```python
from build123d import *

# Parameters (mm, degrees)
SKETCH_1_W                       = 52
SKETCH_1_H                       = 25
SM_BASE_FLANGE_1_DEPTH           = 2
SM_EDGE_FLANGE_1_STRIP_W         = 9.4732
SM_EDGE_FLANGE_1_STRIP_H         = 2
SM_EDGE_FLANGE_1_STRIP_CUT_DEPTH = 25
SM_EDGE_FLANGE_1_DEPTH           = 25
SM_START                         = 2
SM_EDGE_FLANGE_1_FLAT_DEPTH      = 2
HOLE_WIZARD_3_0_3_1_D            = 3
HOLE_WIZARD_8_0_8_2_D            = 8
HOLE_WIZARD_8_0_8_3_D            = 8
HOLE_WIZARD_3_0_3_2_D            = 3


# Sheet-metal steps are written as plain solids
with BuildPart() as part:
    # Sketch 1 → 基体-法兰1 (new body)
    with BuildSketch(Plane(origin=(0, 0, 0), x_dir=(1, 0, 0), z_dir=(0, 1, 0))):
        Rectangle(SKETCH_1_W, SKETCH_1_H)
    extrude(amount=-SM_BASE_FLANGE_1_DEPTH)

    # 边线-法兰1 strip (across the edge) → 边线-法兰1 strip cut (cut)
    with BuildSketch(Plane(origin=(-26, 0, -12.5), x_dir=(1, 0, 0), z_dir=(0, 0, 1))):
        with Locations((-4, -1)):
            Rectangle(SM_EDGE_FLANGE_1_STRIP_W, SM_EDGE_FLANGE_1_STRIP_H)
    sm_edge_flange_1_strip_cut = extrude(amount=SM_EDGE_FLANGE_1_STRIP_CUT_DEPTH, mode=Mode.SUBTRACT)

    # 边线-法兰1 bend section (across the edge) → 边线-法兰1 (add)
    with BuildSketch(Plane(origin=(-26, 0, -12.5), x_dir=(1, 0, 0), z_dir=(0, 0, 1))):
        with BuildLine():
            Line((-2, 0.7366), (0, 0.7366))
            ThreePointArc((0, 0.7366), (0.215745145, 0.215745145), (0.7366, 0))
            Line((0.7366, 0), (0.7366, -2))
            ThreePointArc((0.7366, -2), (-1.198468417, -1.198468417), (-2, 0.7366))
        make_face()
    sm_edge_flange_1 = extrude(amount=SM_EDGE_FLANGE_1_DEPTH)

    # 边线-法兰1 profile (on flange) → 边线-法兰1 flat (add)
    with BuildSketch(Plane.ZY.offset(26).offset(SM_START)):
        with BuildLine():
            ThreePointArc((12.5, 50), (0, 62.5), (-12.5, 50))
            Line((-12.5, 50), (-12.5, 0.7366))
            Line((-12.5, 0.7366), (12.5, 0.7366))
            Line((12.5, 0.7366), (12.5, 50))
        make_face()
    sm_edge_flange_1_flat = extrude(amount=-SM_EDGE_FLANGE_1_FLAT_DEPTH)

    # 镜向1: 边线-法兰1 strip cut, 边线-法兰1, 边线-法兰1 flat across plane
    add(sm_edge_flange_1_strip_cut.mirror(Plane(origin=(0, 0, 0), x_dir=(0, 0, 1), z_dir=(1, 0, 0))), mode=Mode.SUBTRACT)
    add(sm_edge_flange_1.mirror(Plane(origin=(0, 0, 0), x_dir=(0, 0, 1), z_dir=(1, 0, 0))))
    add(sm_edge_flange_1_flat.mirror(Plane(origin=(0, 0, 0), x_dir=(0, 0, 1), z_dir=(1, 0, 0))))

    # Ø3.0 (3) 直径孔1 (through all)
    with Locations(Plane(origin=(0, -2, 0), x_dir=(-1, 0, 0), z_dir=(0, -1, 0))):
        with Locations((0, 7), (0, -7), (7, 0), (18.6, 0), (-7, 0), (-18.6, 0)):
            Hole(HOLE_WIZARD_3_0_3_1_D / 2)

    # Ø8.0 (8) 直径孔2 (through all)
    with Locations(Plane(origin=(0, -2, 0), x_dir=(-1, 0, 0), z_dir=(0, -1, 0))):
        with Locations((0, 0)):
            Hole(HOLE_WIZARD_8_0_8_2_D / 2)

    # Ø8.0 (8) 直径孔3 (through all)
    with Locations(Plane.ZY.offset(28)):
        with Locations((0, 50)):
            Hole(HOLE_WIZARD_8_0_8_3_D / 2)

    # Ø3.0 (3) 直径孔2 (through all)
    with Locations(Plane.ZY.offset(28)):
        with Locations((-7, 50), (7, 50), (0, 57), (0, 43), (0, 31.4), (0, 14.53)):
            Hole(HOLE_WIZARD_3_0_3_2_D / 2)


solid = part.part
```
Design review of the part built by this model. Coordinates are the model's own, in mm. A direction names the side the tool comes from. Coordinates: 2 decimals unless noted, no trailing zeros. Loops run counter-clockwise (first coordinate to the right, second up) from the corner with the lowest first, then second, coordinate; pieces in that order, holes last.
Q1. To check wall thickness, follow line 1 (Z direction, x = 0, y = -1.45); line 2 (X direction, y = 13.5, z = 9.75); line 3 (Y direction, x = 26.9, z = 0). State the ranges of each line that lie inside material, in increasing order.
Reported:
line 1: z = -12.5 to -8.5, -5.5 to -4, 4 to 5.5, 8.5 to 12.5
line 2: x = -28 to -26, 26 to 28
line 3: y = -1.46 to 13.03, 16.03 to 29.9, 32.9 to 41.5, 44.5 to 46, 54 to 55.5, 58.5 to 62.5
Q2. We need section C-C on z = -7. State the section outline as (x, y) points, and give its area (3 significant figures).
Reported:
outline: (-28, 0.74) arc R2.74 ccw to (-25.26, -2) - (-1.5, -2) - (-1.5, 0) - (-25.26, 0) arc R0.74 cw to (-26, 0.74) - (-26, 48.5) - (-28, 48.5) - close; (-28, 51.5) - (-26, 51.5) - (-26, 60.36) - (-28, 60.36) - close; (1.5, -2) - (25.26, -2) arc R2.74 ccw to (28, 0.74) - (28, 48.5) - (26, 48.5) - (26, 0.74) arc R0.74 cw to (25.26, 0) - (1.5, 0) - close; (26, 51.5) - (28, 51.5) - (28, 60.36) - (26, 60.36) - close
area: 332 mm2
Q3. The part is to be moulded in two halves that separate along Y. For faces 1 (the face through (-0.325, -0.986, 8.464)), 2 (the face through (5, 0, 0)), 3 (the face through (-26.986, 41.536, 0.325)), say which applies: +Y half, -Y half, draft (parallel to the pull), parting line (faces both ways), or undercut.
Reported:
face 1: draft
face 2: +Y half
face 3: undercut
Q4. For pin 1 (2.5 mm diameter, centred on y = 57, z = 0, fed in from -X); pin 2 (2 mm diameter, centred on x = 9.5, z = -1, fed in from +Y), all flat-tipped, find the tip position at first contact; note any pin that passes through.
Reported:
pin 1: passes through
pin 2: stops at y = 0
Q5. We need section A-A on x = -7. State the section outline as (y, z) points, and give its area (3 significant figures).
Reported:
outline: (-2, -12.5) - (0, -12.5) - (0, -1.5) - (-2, -1.5) - close; (-2, 1.5) - (0, 1.5) - (0, 12.5) - (-2, 12.5) - close
area: 44.0 mm2
Q6. We need section D-D on y = 31.4. State the section outline as (x, z) points.
Reported:
outline: (-28, -12.5) - (-26, -12.5) - (-26, -1.5) - (-28, -1.5) - close; (-28, 1.5) - (-26, 1.5) - (-26, 12.5) - (-28, 12.5) - close; (26, -12.5) - (28, -12.5) - (28, -1.5) - (26, -1.5) - close; (26, 1.5) - (28, 1.5) - (28, 12.5) - (26, 12.5) - close
Q7. We need section B-B on y = 24.5. State the section outline as (x, z) points, and give its area (3 significant figures).
Reported:
outline: (-28, -12.5) - (-26, -12.5) - (-26, 12.5) - (-28, 12.5) - close; (26, -12.5) - (28, -12.5) - (28, 12.5) - (26, 12.5) - close
area: 100 mm2
Q8. Tool access review of faces 4 (the face through (-26, 32, -3)), 5 (the face through (27.014, 48.536, 7.325)): name each direction out of +Z, -Z, +X, -X, +Y, -Y from which nothing blocks a thin tool from reaching the whole face with its end or side.
Reported:
face 4: +Z, -Z, +Y
face 5: +X, -X
